Verification items for the finished model (mm, model axes). Face numbers are marked on the shaded views. Give positions to 0.01 mm unless a question says otherwise; leave off trailing zeros. Write each loop counter-clockwise with the first axis right and the second up, starting at its lowest first coordinate (ties: lowest second). Pieces come first, ordered by that corner, then holes.
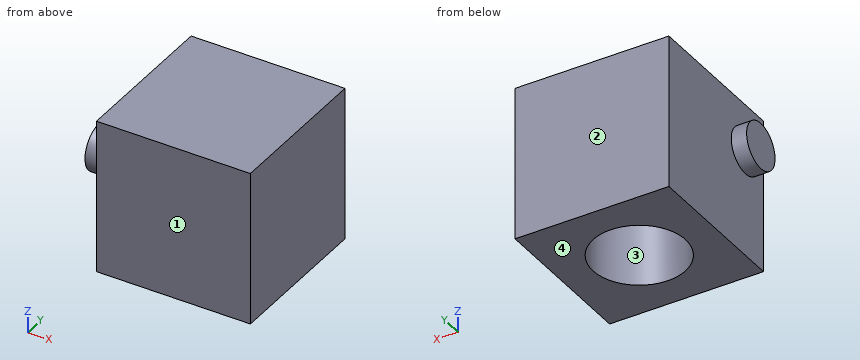
from build123d import *

# Parameters (mm, degrees)
F0_W     = 50
F0_H     = 50
F1_DEPTH = 50
F2_R     = 15
F3_DEPTH = 30
F4_R     = 7.5
F5_DEPTH = 30


with BuildPart() as f1:
    # F0 (on Top) → F1 (new body)
    with BuildSketch(Plane.XY):
        Rectangle(F0_W, F0_H)
    extrude(amount=F1_DEPTH)

    # F2 (on Top) → F3 (cut)
    with BuildSketch(Plane.XY):
        Circle(F2_R)
    extrude(amount=F3_DEPTH, mode=Mode.SUBTRACT)

    # F4 (on Right) → F5 (join)
    with BuildSketch(Plane.YZ):
        with Locations((-15.446586, 34.616902)):
            Circle(F4_R)
    extrude(amount=-F5_DEPTH)


solid = f1.part
Item 1: Scan lines: line 1 along X through (y, z) = (0, 6.5); line 2 along Z through (x, y) = (-3.5, 10). Record each from-to range of solid material in increasing order.
Answer key:
line 1: x = -25 to -15, 15 to 25
line 2: z = 30 to 50
Item 2: Sectioned sample at C-C on x = 14. Record the cut outline in (y, z), then the cut area to 3 significant figures.
Answer key:
outline: (-25, 0) - (-5.39, 0) - (-5.39, 30) - (5.39, 30) - (5.39, 0) - (25, 0) - (25, 50) - (-25, 50) - close
area: 2,180 mm2
Item 3: Depth check by flat-ended pin: pin 1 (6 mm diameter, centred on y = 5, z = 15, fed in from -X). Enter the tip coordinate at first touch or a pass-through.
Answer key:
pin 1: stops at x = -25
Item 4: Release check for a two-part mould opening along Y. For the marked faces 1, 2, 3 and 4 record: released by +Y, released by -Y, zero draft, split by the parting line, or undercut.
Answer key:
face 1: released by -Y
face 2: released by +Y
face 3: undercut
face 4: zero draft
Item 5: Sectioned sample at D-D on y = -14. Record the cut outline in (x, z), then the cut area to 3 significant figures.
Answer key:
outline: (-30, 27.26) - (-25, 27.26) - (-25, 0) - (-5.39, 0) - (-5.39, 27.26) - (0, 27.26) - (0, 30) - (5.39, 30) - (5.39, 0) - (25, 0) - (25, 50) - (-25, 50) - (-25, 41.98) - (-30, 41.98) - close
area: 2,270 mm2
Item 6: Sectioned sample at B-B on y = 0. Record the cut outline in (x, z), then the cut area to 3 significant figures.
Answer key:
outline: (-25, 0) - (-15, 0) - (-15, 30) - (15, 30) - (15, 0) - (25, 0) - (25, 50) - (-25, 50) - close
area: 1,600 mm2
Item 7: Sectioned sample at A-A on z = 23. Record the cut outline in (x, y).
Answer key:
outline: (-25, -25) - (25, -25) - (25, 25) - (-25, 25) - close; hole circle Ø30 at (0, 0)
